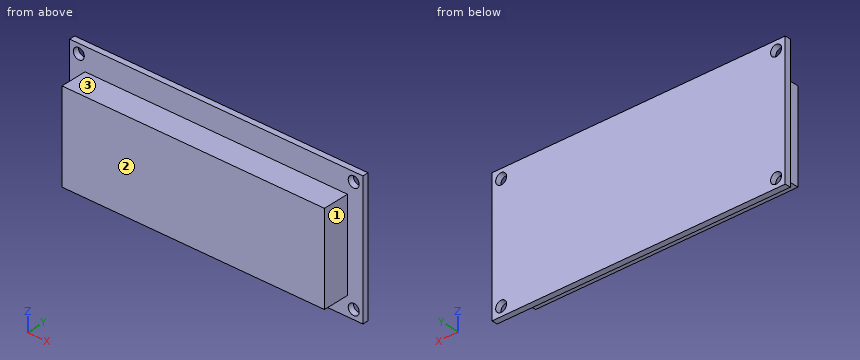
```python
from build123d import *

# Parameters (mm, degrees)
F0_W     = 80
F0_H     = 36
F0_R     = 1.5
F1_DEPTH = 1.6
F2_W     = 71.6
F2_H     = 24.6
F3_DEPTH = 7.2
F4_W     = 65
F4_H     = 14
F5_DEPTH = 1


with BuildPart() as f1:
    # F0 (on Front) → F1 (new body)
    with BuildSketch(Plane.XZ):
        with Locations((2.698481, -4.318948)):
            Rectangle(F0_W, F0_H)
        with Locations((-34.801519, -19.818948)):
            Circle(F0_R, mode=Mode.SUBTRACT)
        with Locations((40.198481, -19.818948)):
            Circle(F0_R, mode=Mode.SUBTRACT)
        with Locations((-34.801519, 11.181052)):
            Circle(F0_R, mode=Mode.SUBTRACT)
        with Locations((40.198481, 11.181052)):
            Circle(F0_R, mode=Mode.SUBTRACT)
    extrude(amount=F1_DEPTH)

    # F2 (on face) → F3 (join)
    with BuildSketch(Plane.XZ.offset(1.6)):
        with Locations((2.698481, -4.818948)):
            Rectangle(F2_W, F2_H)
    extrude(amount=F3_DEPTH)

    # F4 (on face) → F5 (join)
    with BuildSketch(Plane.XZ.offset(8.8)):
        with Locations((2.748481, -5.466159)):
            Rectangle(F4_W, F4_H)
    extrude(amount=-F5_DEPTH)


solid = f1.part
```
Here's how the part is built. I have some questions about the finished solid (model axes, mm). Face numbers are marked on the shaded views. A direction names the side the tool comes from. Coordinates: 2 decimals unless noted, no trailing zeros. Write each loop counter-clockwise with the first axis right and the second up, starting at its lowest first coordinate (ties: lowest second). Pieces come first, ordered by that corner, then holes. Notation, with made-up numbers: M 82.25,8 L 118.25,8 A26 ccw 118.25,36 Z; hole C -1,-17 d3. An arc over 180 degrees is marked long. Answer as CSV lines item,"result". Start each with the question number.
Q1. Suppose I cut it at C-C, the plane y = -2.5. List the corners of the cut face in (x, z) for me.
Q2. Will these pins go through, and if not, where does the flat tip stop? pin 1 Ø3.5 at (y, z) = (-3.5, -6.5) entering from -X; pin 2 Ø1.5 at (y, z) = (-4, -15.5) entering from +X; pin 3 Ø5 at (x, z) = (19, -13.5) entering from +Y; pin 4 Ø4 at (x, z) = (-34.8, 11.18) entering from -Y.
Q3. For the marked faces 1, 2 and 3, which set-ups out of +Z, -Z, +X, -X, +Y, -Y let a thin tool reach every point of the face, with its end or its side?
Q4. Suppose I cut it at D-D, the plane z = 8.5. List the corners of the cut face in (x, y) for me, then the cut area to 3 significant figures.
Q5. Suppose I cut it at B-B, the plane z = -11.5. List the corners of the cut face in (x, y) for me.
Q6. Suppose I cut it at A-A, the plane x = 14. List the corners of the cut face in (y, z) for me.
Q7. I need wall thicknesses on probe 1 along Z at (x, y) = (21, -4.25); probe 2 along X at (y, z) = (-3.5, -8); probe 3 along Y at (x, z) = (-10.5, 9). Which ranges of each line are inside material? Lowest first, please. Write a range as [from, to].
Entries:
1,outline,"M -33.1,-17.12 L 38.5,-17.12 L 38.5,7.48 L -33.1,7.48 Z"
2,pin 1,"stops at x = -33.1"
2,pin 2,"stops at x = 38.5"
2,pin 3,"stops at y = 0"
2,pin 4,"stops at y = -1.6"
3,face 1,"+Z, -Z, +X, -Y"
3,face 2,"+Z, -Z, +X, -X, -Y"
3,face 3,"+Z, +X, -X, -Y"
4,outline,"M -37.3,-1.6 L 42.7,-1.6 L 42.7,0 L -37.3,0 Z"
4,area,"128 mm²"
5,outline,"M -37.3,-1.6 L -33.1,-1.6 L -33.1,-8.8 L 38.5,-8.8 L 38.5,-1.6 L 42.7,-1.6 L 42.7,0 L -37.3,0 Z"
6,outline,"M -8.8,-17.12 L -1.6,-17.12 L -1.6,-22.32 L 0,-22.32 L 0,13.68 L -1.6,13.68 L -1.6,7.48 L -8.8,7.48 Z"
7,probe 1,"z = [-17.12, 7.48]"
7,probe 2,"x = [-33.1, 38.5]"
7,probe 3,"y = [-1.6, 0]"
